Work out the finished part from the listing and answer in its coordinate system (mm). A direction names the side the tool comes from. Round coordinates to 2 decimals unless told otherwise and drop trailing zeros. Order: outer loops, then holes, each group sorted by start corner. A loop starts at its lowest first (then second) coordinate and runs counter-clockwise, first axis right, second up. Notation, with made-up numbers: (-6, 25.5) - (21, 25.5) arc R22 ccw to (21, 53.5) - close; hole circle Ø9 at (58.5, 59.5). An arc over 180 degrees is marked (long way). Answer in a Markdown table with one row per item.
from build123d import *

# Parameters (mm, degrees)
F1_DEPTH = 25.4
F3_DEPTH = 44.45
F5_DEPTH = 57.15
F6_R     = 25.4
F7_DEPTH = 177.8


with BuildPart() as f1:
    # F0 (on Top) → F1 (new body)
    with BuildSketch(Plane.XY):
        with BuildLine():
            ThreePointArc((-38.1, 0), (-37.551305, 6.442785), (-35.921024, 12.7))
            Line((-35.921024, 12.7), (-69.85, 0))
            Line((-69.85, 0), (-38.1, 0))
        make_face()
        with BuildLine():
            Line((-69.85, 0), (-35.921024, -12.7))
            ThreePointArc((-35.921024, -12.7), (-37.551305, -6.442785), (-38.1, 0))
            Line((-38.1, 0), (-69.85, 0))
        make_face()
        with BuildLine():
            ThreePointArc((35.921024, 12.7), (37.551305, 6.442785), (38.1, 0))
            ThreePointArc((38.1, 0), (37.551305, -6.442785), (35.921024, -12.7))
            Line((35.921024, -12.7), (69.85, 0))
            Line((69.85, 0), (35.921024, 12.7))
        make_face()
        with BuildLine():
            ThreePointArc((0, 38.1), (6.442785, 37.551305), (12.7, 35.921024))
            Line((12.7, 35.921024), (0, 69.85))
            Line((0, 69.85), (0, 38.1))
        make_face()
        with BuildLine():
            ThreePointArc((-12.7, 35.921024), (-6.442785, 37.551305), (0, 38.1))
            Line((0, 38.1), (0, 69.85))
            Line((0, 69.85), (-12.7, 35.921024))
        make_face()
        with BuildLine():
            ThreePointArc((35.921024, -12.7), (37.551305, -6.442785), (38.1, 0))
            ThreePointArc((38.1, 0), (37.551305, 6.442785), (35.921024, 12.7))
            ThreePointArc((35.921024, 12.7), (26.940768, 26.940768), (12.7, 35.921024))
            ThreePointArc((12.7, 35.921024), (6.442785, 37.551305), (0, 38.1))
            ThreePointArc((0, 38.1), (-6.442785, 37.551305), (-12.7, 35.921024))
            ThreePointArc((-12.7, 35.921024), (-26.940768, 26.940768), (-35.921024, 12.7))
            ThreePointArc((-35.921024, 12.7), (-37.551305, 6.442785), (-38.1, 0))
            ThreePointArc((-38.1, 0), (-37.551305, -6.442785), (-35.921024, -12.7))
            ThreePointArc((-35.921024, -12.7), (-26.940768, -26.940768), (-12.7, -35.921024))
            ThreePointArc((-12.7, -35.921024), (0, -38.1), (12.7, -35.921024))
            ThreePointArc((12.7, -35.921024), (26.940768, -26.940768), (35.921024, -12.7))
        make_face()
        with BuildLine():
            Line((0, -69.85), (12.7, -35.921024))
            ThreePointArc((12.7, -35.921024), (0, -38.1), (-12.7, -35.921024))
            Line((-12.7, -35.921024), (0, -69.85))
        make_face()
    extrude(amount=F1_DEPTH)

    # F2 (on Top) → F3 (join)
    with BuildSketch(Plane.XY):
        with BuildLine():
            ThreePointArc((30.28757, -9.525), (31.382263, -4.818307), (31.75, 0))
            ThreePointArc((31.75, 0), (31.382263, 4.818307), (30.28757, 9.525))
            ThreePointArc((30.28757, 9.525), (22.45064, 22.45064), (9.525, 30.28757))
            ThreePointArc((9.525, 30.28757), (0, 31.75), (-9.525, 30.28757))
            ThreePointArc((-9.525, 30.28757), (-22.45064, 22.45064), (-30.28757, 9.525))
            ThreePointArc((-30.28757, 9.525), (-31.382263, 4.818307), (-31.75, 0))
            ThreePointArc((-31.75, 0), (-31.382263, -4.818307), (-30.28757, -9.525))
            ThreePointArc((-30.28757, -9.525), (-22.45064, -22.45064), (-9.525, -30.28757))
            ThreePointArc((-9.525, -30.28757), (-4.818307, -31.382263), (0, -31.75))
            ThreePointArc((0, -31.75), (4.818307, -31.382263), (9.525, -30.28757))
            ThreePointArc((9.525, -30.28757), (22.45064, -22.45064), (30.28757, -9.525))
        make_face()
        with BuildLine():
            ThreePointArc((30.28757, 9.525), (31.382263, 4.818307), (31.75, 0))
            ThreePointArc((31.75, 0), (31.382263, -4.818307), (30.28757, -9.525))
            Line((30.28757, -9.525), (57.15, 0))
            Line((57.15, 0), (30.28757, 9.525))
        make_face()
        with BuildLine():
            ThreePointArc((-9.525, 30.28757), (0, 31.75), (9.525, 30.28757))
            Line((9.525, 30.28757), (0, 57.15))
            Line((0, 57.15), (-9.525, 30.28757))
        make_face()
        with BuildLine():
            Line((0, -57.15), (9.525, -30.28757))
            ThreePointArc((9.525, -30.28757), (4.818307, -31.382263), (0, -31.75))
            Line((0, -31.75), (0, -57.15))
        make_face()
        with BuildLine():
            Line((0, -57.15), (0, -31.75))
            ThreePointArc((0, -31.75), (-4.818307, -31.382263), (-9.525, -30.28757))
            Line((-9.525, -30.28757), (0, -57.15))
        make_face()
        with BuildLine():
            ThreePointArc((-31.75, 0), (-31.382263, 4.818307), (-30.28757, 9.525))
            Line((-30.28757, 9.525), (-57.15, 0))
            Line((-57.15, 0), (-31.75, 0))
        make_face()
        with BuildLine():
            ThreePointArc((-30.28757, -9.525), (-31.382263, -4.818307), (-31.75, 0))
            Line((-31.75, 0), (-57.15, 0))
            Line((-57.15, 0), (-30.28757, -9.525))
        make_face()
    extrude(amount=F3_DEPTH)

    # F4 (on Top) → F5 (join)
    with BuildSketch(Plane.XY):
        with BuildLine():
            ThreePointArc((24.593444, -6.35), (25.197554, -3.200509), (25.4, 0))
            ThreePointArc((25.4, 0), (25.197554, 3.200509), (24.593444, 6.35))
            ThreePointArc((24.593444, 6.35), (17.960512, 17.960512), (6.35, 24.593444))
            ThreePointArc((6.35, 24.593444), (3.200509, 25.197554), (0, 25.4))
            ThreePointArc((0, 25.4), (-3.200509, 25.197554), (-6.35, 24.593444))
            ThreePointArc((-6.35, 24.593444), (-17.960512, 17.960512), (-24.593444, 6.35))
            ThreePointArc((-24.593444, 6.35), (-25.197554, 3.200509), (-25.4, 0))
            ThreePointArc((-25.4, 0), (-25.197554, -3.200509), (-24.593444, -6.35))
            ThreePointArc((-24.593444, -6.35), (-17.960512, -17.960512), (-6.35, -24.593444))
            ThreePointArc((-6.35, -24.593444), (0, -25.4), (6.35, -24.593444))
            ThreePointArc((6.35, -24.593444), (17.960512, -17.960512), (24.593444, -6.35))
        make_face()
        with BuildLine():
            ThreePointArc((24.593444, 6.35), (25.197554, 3.200509), (25.4, 0))
            ThreePointArc((25.4, 0), (25.197554, -3.200509), (24.593444, -6.35))
            Line((24.593444, -6.35), (44.45, 0))
            Line((44.45, 0), (24.593444, 6.35))
        make_face()
        with BuildLine():
            ThreePointArc((0, 25.4), (3.200509, 25.197554), (6.35, 24.593444))
            Line((6.35, 24.593444), (0, 44.45))
            Line((0, 44.45), (0, 25.4))
        make_face()
        with BuildLine():
            Line((0, -44.45), (6.35, -24.593444))
            ThreePointArc((6.35, -24.593444), (0, -25.4), (-6.35, -24.593444))
            Line((-6.35, -24.593444), (0, -44.45))
        make_face()
        with BuildLine():
            ThreePointArc((-6.35, 24.593444), (-3.200509, 25.197554), (0, 25.4))
            Line((0, 25.4), (0, 44.45))
            Line((0, 44.45), (-6.35, 24.593444))
        make_face()
        with BuildLine():
            Line((-44.45, 0), (-24.593444, -6.35))
            ThreePointArc((-24.593444, -6.35), (-25.197554, -3.200509), (-25.4, 0))
            Line((-25.4, 0), (-44.45, 0))
        make_face()
        with BuildLine():
            ThreePointArc((-25.4, 0), (-25.197554, 3.200509), (-24.593444, 6.35))
            Line((-24.593444, 6.35), (-44.45, 0))
            Line((-44.45, 0), (-25.4, 0))
        make_face()
    extrude(amount=F5_DEPTH)

    # F6 (on Top) → F7 (join)
    with BuildSketch(Plane.XY):
        Circle(F6_R)
    extrude(amount=F7_DEPTH)


solid = f1.part
1) Find the intervals of material crossed by probe 1 along Z at (x, y) = (-3, 39); probe 2 along Y at (x, z) = (0, 119.5); probe 3 along Z at (x, y) = (57.5, -4.5), in increasing order. Write a range as from..to.
Filled in:
| item | result |
|---|---|
| probe 1 | z = 0..44.45 |
| probe 2 | y = -25.4..25.4 |
| probe 3 | z = 0..25.4 |
2) Which of the six approach directions +Z, -Z, +X, -X, +Y, -Y give full straight-line access (tool end or side, diameter ignored) to faces 1 (the face through (43.9, 4.7, 34.8)), 2 (the face through (-6.261, 53.123, 12.522)), 3 (the face through (-34.38, 3.22, 50.71)), 4 (the face through (-22.6, -22.3, 34.8)), 5 (the face through (-53.123, -6.261, 12.522))?
Filled in:
| item | result |
|---|---|
| face 1 | +Z, +X, +Y |
| face 2 | +Z, -Z, -X, +Y |
| face 3 | +Z, -X, +Y |
| face 4 | +Z, -X, -Y |
| face 5 | +Z, -Z, -X, -Y |
3) Find section C-C, the plane x = -61. Give the vertices of the cut face in (y, z), then the cut area to 3 significant figures.
Filled in:
| item | result |
|---|---|
| outline | (-3.31, 0) - (3.31, 0) - (3.31, 25.4) - (-3.31, 25.4) - close |
| area | 168 mm^2 |
4) Find section A-A, the plane z = 55. Give the vertices of the cut face in (x, y).
Filled in:
| item | result |
|---|---|
| outline | (-44.45, 0) - (-24.59, -6.35) arc R25.4 ccw to (-6.35, -24.59) - (0, -44.45) - (6.35, -24.59) arc R25.4 ccw to (24.59, -6.35) - (44.45, 0) - (24.59, 6.35) arc R25.4 ccw to (6.35, 24.59) - (0, 44.45) - (-6.35, 24.59) arc R25.4 ccw to (-24.59, 6.35) - close |
5) Find section B-B, the plane y = 18. Give the vertices of the cut face in (x, z).
Filled in:
| item | result |
|---|---|
| outline | (-33.58, 0) - (33.58, 0) - (33.58, 25.4) - (26.15, 25.4) - (26.15, 44.45) - (17.92, 44.45) - (17.92, 177.8) - (-17.92, 177.8) - (-17.92, 44.45) - (-26.15, 44.45) - (-26.15, 25.4) - (-33.58, 25.4) - close |
6) Each of these flat-tipped pins is pushed along its axis until it touches: pin 1 (8 mm diameter, centred on x = -20, z = 127.5, fed in from +Y); pin 2 (6 mm diameter, centred on x = 53.5, z = 43, fed in from +Y); pin 3 (10 mm diameter, centred on x = 37.5, y = -1, fed in from +Z). Where does it stop, or does it pass through?
Filled in:
| item | result |
|---|---|
| pin 1 | stops at y = 19.73 |
| pin 2 | stops at y = 2.36 |
| pin 3 | stops at z = 57.15 |
